Check sheet for the modelled part. Datum: model origin and axes. Units: mm. A direction names the side the tool comes from. Give positions to 0.01 mm unless a question says otherwise; leave off trailing zeros. Order: outer loops, then holes, each group sorted by start corner. A loop starts at its lowest first (then second) coordinate and runs counter-clockwise, first axis right, second up. Notation, with made-up numbers: (21.5, 73) -> (74.5, 73) arc R30 ccw to (74.5, 105) -> close; hole circle Ø10 at (15.25, -22.75). An arc over 180 degrees is marked (long way). Answer in a Markdown table with one row per item. Add a question column.
(1) Release check for a two-part mould opening along X. For faces 4 (the face through (60, -27, 2)), 5 (the face through (82.5, 0, 2)), 6 (the face through (-43.5, 0, 2)), 7 (the face through (35, -31, 2)) record: released by +X, released by -X, zero draft, split by the parting line, or undercut.
(2) Set-up check for faces 1 (the face through (-60, -27, 2)), 2 (the face through (46.5, 0, 2)), 3 (the face through (-1, 8, 0)): record each of +Z, -Z, +X, -X, +Y, -Y from which the full face is reachable in a straight line by a thin tool's end or side.
(3) Cross-section at D-D (y = 3.5). Record the cut outline in (x, z), then the cut area to 3 significant figures.
(4) Thickness scan on L1, parallel to Y at x = 14.5, z = 2.75; L2, parallel to Y at x = 6, z = 1.9; L3, parallel to Y at x = -18.5, z = 2.05. Record the ranges inside material, lowest first. Write a range as [from, to].
(5) Cross-section at B-B (x = 81). Record the cut outline in (y, z), then the cut area to 3 significant figures.
(6) Cross-section at A-A (x = -17). Record the cut outline in (y, z).
(7) Go/stop test with a flat-tipped pin: pin 1 (0.9 mm diameter, centred on y = 31.5, z = 1.5, fed in from +X). Record where the tip stops, or that it passes through.
(8) Cross-section at C-C (x = 18). Record the cut outline in (y, z), then the cut area to 3 significant figures.
```python
from build123d import *

# Parameters (mm, degrees)
SKETCH_1_W          = 170
SKETCH_1_H          = 70
EXTRUDE_1_DEPTH     = 3
SKETCH_2_R          = 5
SKETCH_2_R_2        = 1.1
CUT_EXTRUDE_1_DEPTH = 92.972822073
CUT_EXTRUDE_2_DEPTH = 92.972822073


with BuildPart() as part:
    # 草圖1 → 填料-伸長1 (new body)
    with BuildSketch(Plane.XY):
        Rectangle(SKETCH_1_W, SKETCH_1_H)
    extrude(amount=EXTRUDE_1_DEPTH)

    # 草圖2 → 除料-伸長1 (cut, through all)
    with BuildSketch(Plane.XY.offset(3)):
        Circle(SKETCH_2_R)
        with Locations((27, -20.5)):
            Circle(SKETCH_2_R_2)
        with Locations((6, -20.5)):
            Circle(SKETCH_2_R_2)
        with Locations((6, -33)):
            Circle(SKETCH_2_R_2)
        with Locations((27, -33)):
            Circle(SKETCH_2_R_2)
        with BuildLine():
            Line((43.5, -22.5), (43.5, 22.5))
            ThreePointArc((43.5, 22.5), (45, 24), (46.5, 22.5))
            Line((46.5, 22.5), (46.5, -22.5))
            ThreePointArc((46.5, -22.5), (45, -24), (43.5, -22.5))
        make_face()
        with BuildLine():
            Line((-46.5, -22.5), (-46.5, 22.5))
            ThreePointArc((-46.5, 22.5), (-45, 24), (-43.5, 22.5))
            Line((-43.5, 22.5), (-43.5, -22.5))
            ThreePointArc((-43.5, -22.5), (-45, -24), (-46.5, -22.5))
        make_face()
        with BuildLine():
            Line((-82.5, -22.5), (-82.5, 22.5))
            ThreePointArc((-82.5, 22.5), (-81, 24), (-79.5, 22.5))
            Line((-79.5, 22.5), (-79.5, -22.5))
            ThreePointArc((-79.5, -22.5), (-81, -24), (-82.5, -22.5))
        make_face()
        with BuildLine():
            Line((79.5, -22.5), (79.5, 22.5))
            ThreePointArc((79.5, 22.5), (81, 24), (82.5, 22.5))
            Line((82.5, 22.5), (82.5, -22.5))
            ThreePointArc((82.5, -22.5), (81, -24), (79.5, -22.5))
        make_face()
        with BuildLine():
            Line((21.5, -31.5), (8.5, -31.5))
            ThreePointArc((8.5, -31.5), (7, -30), (8.5, -28.5))
            Line((8.5, -28.5), (21.5, -28.5))
            ThreePointArc((21.5, -28.5), (23, -30), (21.5, -31.5))
        make_face()
        with BuildLine():
            Line((-21.5, -31.5), (-8.5, -31.5))
            ThreePointArc((-8.5, -31.5), (-7, -30), (-8.5, -28.5))
            Line((-8.5, -28.5), (-21.5, -28.5))
            ThreePointArc((-21.5, -28.5), (-23, -30), (-21.5, -31.5))
        make_face()
        with BuildLine():
            Line((21.5, 31.5), (8.5, 31.5))
            ThreePointArc((8.5, 31.5), (7, 30), (8.5, 28.5))
            Line((8.5, 28.5), (21.5, 28.5))
            ThreePointArc((21.5, 28.5), (23, 30), (21.5, 31.5))
        make_face()
        with BuildLine():
            Line((-21.5, 31.5), (-8.5, 31.5))
            ThreePointArc((-8.5, 31.5), (-7, 30), (-8.5, 28.5))
            Line((-8.5, 28.5), (-21.5, 28.5))
            ThreePointArc((-21.5, 28.5), (-23, 30), (-21.5, 31.5))
        make_face()
        with BuildLine():
            Line((21.5, 24), (8.5, 24))
            ThreePointArc((8.5, 24), (7, 22.5), (8.5, 21))
            Line((8.5, 21), (21.5, 21))
            ThreePointArc((21.5, 21), (23, 22.5), (21.5, 24))
        make_face()
        with BuildLine():
            Line((-21.5, 24), (-8.5, 24))
            ThreePointArc((-8.5, 24), (-7, 22.5), (-8.5, 21))
            Line((-8.5, 21), (-21.5, 21))
            ThreePointArc((-21.5, 21), (-23, 22.5), (-21.5, 24))
        make_face()
        with BuildLine():
            Line((-21.5, -24), (-8.5, -24))
            ThreePointArc((-8.5, -24), (-7, -22.5), (-8.5, -21))
            Line((-8.5, -21), (-21.5, -21))
            ThreePointArc((-21.5, -21), (-23, -22.5), (-21.5, -24))
        make_face()
    extrude(amount=-CUT_EXTRUDE_1_DEPTH, mode=Mode.SUBTRACT)

    # 草圖4 → 除料-伸長2 (cut, through all)
    with BuildSketch(Plane.XY.offset(3)):
        with BuildLine():
            Line((85, 35), (35, 35))
            Line((35, 35), (33, 35))
            ThreePointArc((33, 35), (34.414213562, 34.414213562), (35, 33))
            Line((35, 33), (35, 29))
            ThreePointArc((35, 29), (35.585786438, 27.585786438), (37, 27))
            Line((37, 27), (83, 27))
            ThreePointArc((83, 27), (84.414213562, 26.414213562), (85, 25))
            Line((85, 25), (85, 27))
            Line((85, 27), (85, 35))
        make_face()
        with BuildLine():
            Line((85, -27), (85, -25))
            ThreePointArc((85, -25), (84.414213562, -26.414213562), (83, -27))
            Line((83, -27), (37, -27))
            ThreePointArc((37, -27), (35.585786438, -27.585786438), (35, -29))
            Line((35, -29), (35, -33))
            ThreePointArc((35, -33), (34.414213562, -34.414213562), (33, -35))
            Line((33, -35), (35, -35))
            Line((35, -35), (85, -35))
            Line((85, -35), (85, -27))
        make_face()
        with BuildLine():
            Line((-85, -35), (-35, -35))
            Line((-35, -35), (-33, -35))
            ThreePointArc((-33, -35), (-34.414213562, -34.414213562), (-35, -33))
            Line((-35, -33), (-35, -29))
            ThreePointArc((-35, -29), (-35.585786438, -27.585786438), (-37, -27))
            Line((-37, -27), (-83, -27))
            ThreePointArc((-83, -27), (-84.414213562, -26.414213562), (-85, -25))
            Line((-85, -25), (-85, -27))
            Line((-85, -27), (-85, -35))
        make_face()
        with BuildLine():
            Line((-85, 27), (-85, 25))
            ThreePointArc((-85, 25), (-84.414213562, 26.414213562), (-83, 27))
            Line((-83, 27), (-37, 27))
            ThreePointArc((-37, 27), (-35.585786438, 27.585786438), (-35, 29))
            Line((-35, 29), (-35, 33))
            ThreePointArc((-35, 33), (-34.414213562, 34.414213562), (-33, 35))
            Line((-33, 35), (-35, 35))
            Line((-35, 35), (-85, 35))
            Line((-85, 35), (-85, 27))
        make_face()
    extrude(amount=-CUT_EXTRUDE_2_DEPTH, mode=Mode.SUBTRACT)


solid = part.part
```
Answer below:
| question | item | result |
|---|---|---|
| 1 | face 4 | zero draft |
| 1 | face 5 | undercut |
| 1 | face 6 | undercut |
| 1 | face 7 | released by +X |
| 2 | face 1 | +Z, -Z, -X, -Y |
| 2 | face 2 | +Z, -Z |
| 2 | face 3 | -Z, +X, -X, +Y, -Y |
| 3 | outline | (-85, 0) -> (-82.5, 0) -> (-82.5, 3) -> (-85, 3) -> close; (-79.5, 0) -> (-46.5, 0) -> (-46.5, 3) -> (-79.5, 3) -> close; (-43.5, 0) -> (-3.57, 0) -> (-3.57, 3) -> (-43.5, 3) -> close; (3.57, 0) -> (43.5, 0) -> (43.5, 3) -> (3.57, 3) -> close; (46.5, 0) -> (79.5, 0) -> (79.5, 3) -> (46.5, 3) -> close; (82.5, 0) -> (85, 0) -> (85, 3) -> (82.5, 3) -> close |
| 3 | area | 453 mm² |
| 4 | L1 | y = [-35, -31.5], [-28.5, 21], [24, 28.5], [31.5, 35] |
| 4 | L2 | y = [-35, -34.1], [-31.9, -21.6], [-19.4, 35] |
| 4 | L3 | y = [-35, -31.5], [-28.5, -24], [-21, 21], [24, 28.5], [31.5, 35] |
| 5 | outline | (-27, 0) -> (-24, 0) -> (-24, 3) -> (-27, 3) -> close; (24, 0) -> (27, 0) -> (27, 3) -> (24, 3) -> close |
| 5 | area | 18.0 mm² |
| 6 | outline | (-35, 0) -> (-31.5, 0) -> (-31.5, 3) -> (-35, 3) -> close; (-28.5, 0) -> (-24, 0) -> (-24, 3) -> (-28.5, 3) -> close; (-21, 0) -> (21, 0) -> (21, 3) -> (-21, 3) -> close; (24, 0) -> (28.5, 0) -> (28.5, 3) -> (24, 3) -> close; (31.5, 0) -> (35, 0) -> (35, 3) -> (31.5, 3) -> close |
| 7 | pin 1 | stops at x = 35 |
| 8 | outline | (-35, 0) -> (-31.5, 0) -> (-31.5, 3) -> (-35, 3) -> close; (-28.5, 0) -> (21, 0) -> (21, 3) -> (-28.5, 3) -> close; (24, 0) -> (28.5, 0) -> (28.5, 3) -> (24, 3) -> close; (31.5, 0) -> (35, 0) -> (35, 3) -> (31.5, 3) -> close |
| 8 | area | 183 mm² |
